Input: dimensioned drawing with shaded views. Units: mm. Origin: part minimum x, y, z. A direction names the side the tool comes from. Give positions to 0.01 mm unless a question says otherwise; leave off trailing zeros. Loops run counter-clockwise (first coordinate to the right, second up) from the corner with the lowest first, then second, coordinate; pieces in that order, holes last. Notation, with made-up numbers: M 1.25,65 L 53.25,65 A26 ccw 53.25,90 Z; hole C -24.5,89.5 d9. An arc over 180 degrees is marked long. Use CSV: the item, a comma, the result in double quotes. Start each with the question number.
Q1. Pull-direction query (X, two-part tool) for the marked faces 1 and 2; classes: released by +X, released by -X, zero draft, split by the parting line, or undercut.
Q2. Section C-C, the plane x = 1.8. Output: boundary loops of the cut face in (y, z), plus the area to 3 significant figures.
Q3. Section D-D, the plane x = 4.7. Output: boundary loops of the cut face in (y, z), plus the area to 3 significant figures.
Q4. Pin query (flat end, axial travel): pin 1 (1 mm diameter, centred on x = 2.5, z = 4, fed in from -Y) (3 decimals); pin 2 (2 mm diameter, centred on x = 1, y = 1, fed in from +Z). Return the tip coordinate at first contact, or that it passes through.
Q5. Section A-A, the plane y = 0.5. Output: boundary loops of the cut face in (x, z), plus the area to 3 significant figures.
Q6. Section B-B, the plane z = 3.7. Output: boundary loops of the cut face in (x, y), plus the area to 3 significant figures.
Q7. Reachability of the marked faces 3 and 4 from +Z, -Z, +X, -X, +Y, -Y: full face, straight path, thin tool, end or side. Return the list, or none.
Q8. Material intervals for line 1 along X through (y, z) = (3, 1.3); line 2 along X through (y, z) = (3, 2.95); line 3 along Z through (x, y) = (3.6, 6), sorted ascending.
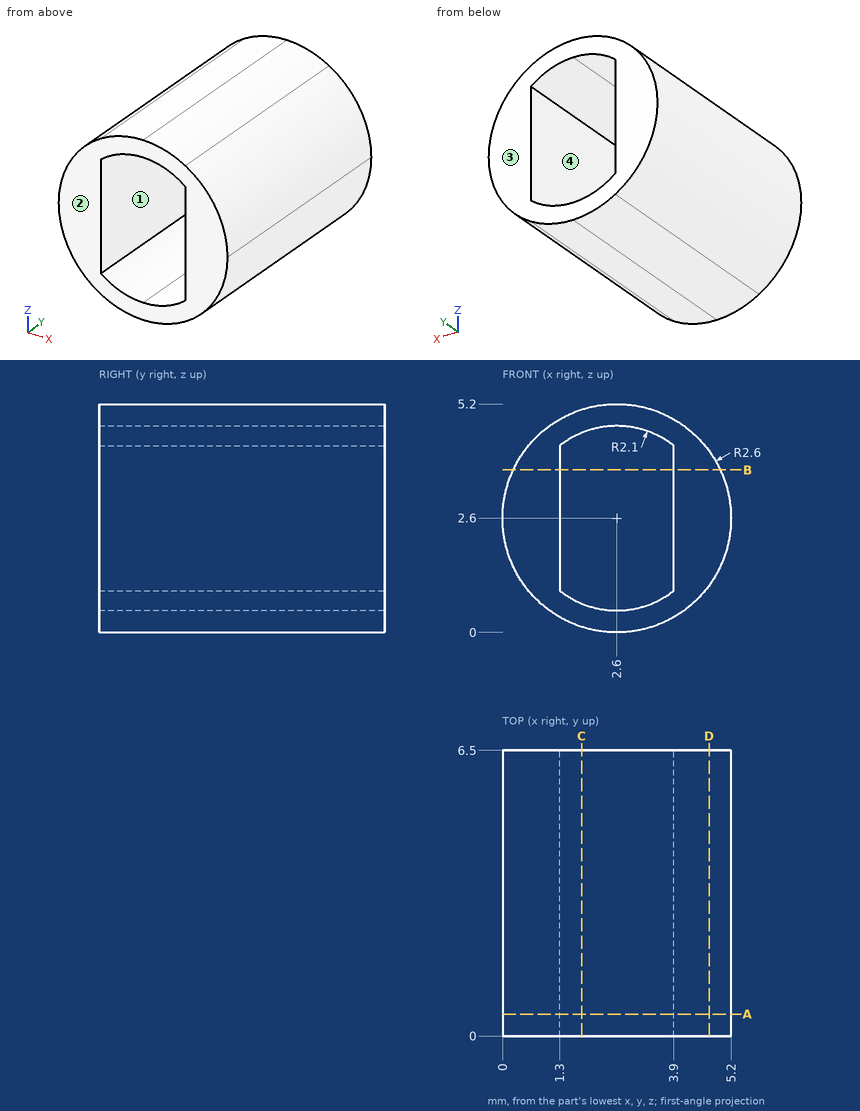
A:
1,face 1,"undercut"
1,face 2,"zero draft"
2,outline,"M 0,0.13 L 6.5,0.13 L 6.5,0.66 L 0,0.66 Z; M 0,4.54 L 6.5,4.54 L 6.5,5.07 L 0,5.07 Z"
2,area,"6.92 mm^2"
3,outline,"M 0,1.07 L 6.5,1.07 L 6.5,4.13 L 0,4.13 Z"
3,area,"19.9 mm^2"
4,pin 1,"through"
4,pin 2,"z = 5.13"
5,outline,"C 2.6,2.6 d5.2; hole M 1.3,0.95 A2.1 ccw 3.9,0.95 L 3.9,4.25 A2.1 ccw 1.3,4.25 Z"
5,area,"11.1 mm^2"
6,outline,"M 0.24,0 L 1.3,0 L 1.3,6.5 L 0.24,6.5 Z; M 3.9,0 L 4.96,0 L 4.96,6.5 L 3.9,6.5 Z"
6,area,"13.7 mm^2"
7,face 3,"+Z, -Z, +X, -X, +Y"
7,face 4,"+Y, -Y"
8,line 1,"0.35 to 1.3, 3.9 to 4.85"
8,line 2,"0.02 to 1.3, 3.9 to 5.18"
8,line 3,"0.2 to 0.75, 4.45 to 5"
